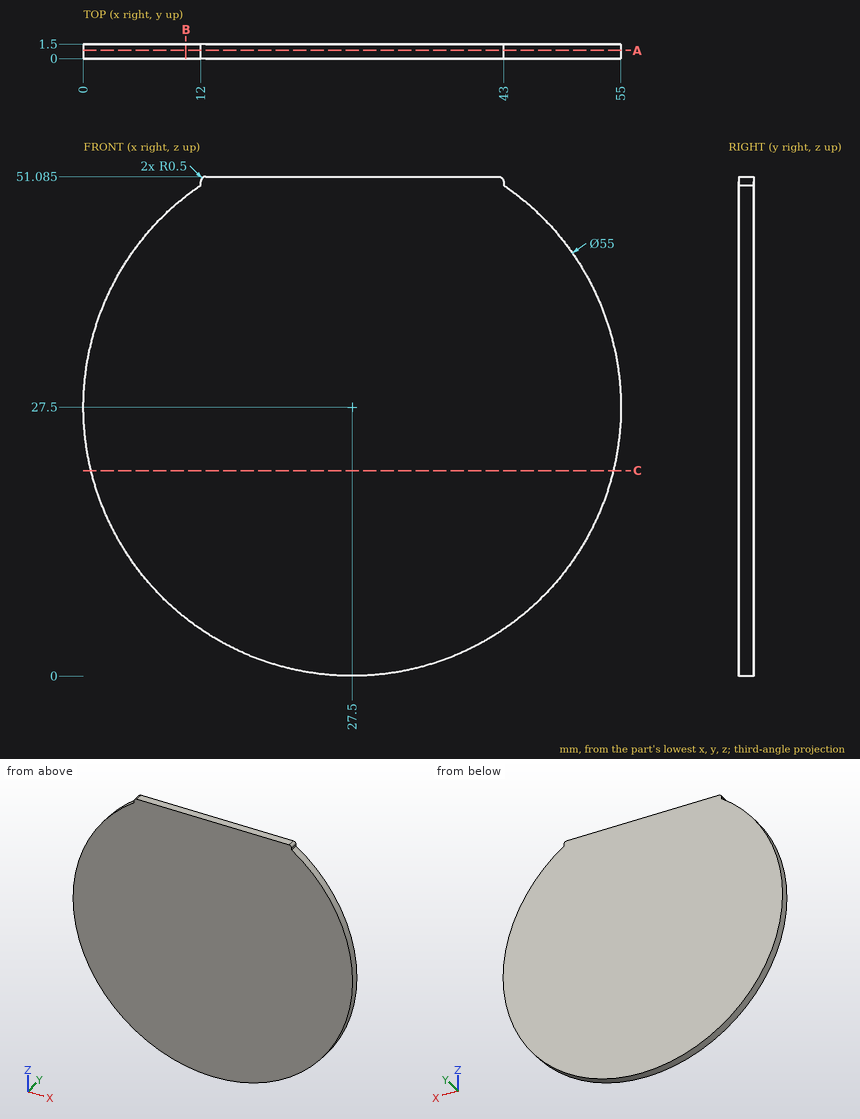
Verification items for this drawing (mm, ordinates from the low corner). Give positions to 0.01 mm unless a question says otherwise; leave off trailing zeros. Loops run counter-clockwise (first coordinate to the right, second up) from the corner with the lowest first, then second, coordinate; pieces in that order, holes last. Notation, with made-up numbers: M -18.5,87.25 L 10.5,87.25 A6 ccw 10.5,91.25 Z; hole C -6,49 d3. An arc over 180 degrees is marked long. Answer in a Markdown table with one row per item.
1) Thickness scan on line 1 (X direction, y = 1.3, z = 35); line 2 (Z direction, x = 16, y = 1.4) (3 decimals); line 3 (X direction, y = 1.15, z = 12). Record the ranges inside material, lowest first.
Solutions:
| item | result |
|---|---|
| line 1 | x = 1.04 to 53.96 |
| line 2 | z = 2.52 to 51.085 |
| line 3 | x = 4.78 to 50.22 |
2) Cross-section at C-C (z = 21). Enter the section's corners in (x, y), plus the area to 3 significant figures.
Solutions:
| item | result |
|---|---|
| outline | M 0.78,0 L 54.22,0 L 54.22,1.5 L 0.78,1.5 Z |
| area | 80.2 mm^2 |
3) Cross-section at A-A (y = 0.85). Enter the section's corners in (x, z) (3 decimals), plus the area to 3 significant figures.
Solutions:
| item | result |
|---|---|
| outline | M 12,50.216 A27.5 ccw long 43,50.216 L 43,50.585 A0.5 ccw 42.5,51.085 L 12.5,51.085 A0.5 ccw 12,50.585 Z |
| area | 2,300 mm^2 |
4) Cross-section at B-B (x = 10.5). Enter the section's corners in (y, z).
Solutions:
| item | result |
|---|---|
| outline | M 0,5.88 L 1.5,5.88 L 1.5,49.12 L 0,49.12 Z |
